CAD build for the part. Positions are in the model's coordinates, mm. A direction names the side the tool comes from. Round coordinates to 2 decimals unless told otherwise and drop trailing zeros. Write each loop counter-clockwise with the first axis right and the second up, starting at its lowest first coordinate (ties: lowest second). Pieces come first, ordered by that corner, then holes. Notation, with made-up numbers: M 82.5,35 L 114.5,35 A27 ccw 114.5,59 Z; hole C 71,-19.75 d10. An arc over 180 degrees is marked long. Write each question's results on one line, items separated by ' | '. Start each with the question number.
```python
from build123d import *

# Parameters (mm, degrees)
SKETCH1_R           = 2.1
SKETCH1_R_2         = 2.85
BOSS_EXTRUDE1_DEPTH = 9
CUT_EXTRUDE1_DEPTH  = 4
SKETCH10_W          = 28.2
SKETCH10_H          = 42
CUT_EXTRUDE8_DEPTH  = 5
SKETCH11_R          = 2.1
CUT_EXTRUDE9_DEPTH  = 5
CUT_EXTRUDE2_DEPTH  = 2
SKETCH5_R           = 2.85
CUT_EXTRUDE3_DEPTH  = 8
SKETCH7_W           = 75.2
SKETCH7_H           = 40.5
CUT_EXTRUDE5_DEPTH  = 6
SKETCH12_R          = 2.85
CUT_EXTRUDE10_DEPTH = 10
CUT_EXTRUDE11_DEPTH = 0.9
FILLET1_R           = 2
FILLET2_R           = 2
FILLET3_R           = 2


with BuildPart() as part:
    # Sketch1 → Boss-Extrude1 (new body)
    with BuildSketch(Plane(origin=(0, 0, 0), x_dir=(1, 0, 0), z_dir=(0, 1, 0))):
        Polygon((76.6, 0), (125, 0), (125, 150), (0, 150), (0, 0), (48.4, 0), (48.4, -15), (76.6, -15), align=None)
        with Locations((6.1, 127.9)):
            Circle(SKETCH1_R, mode=Mode.SUBTRACT)
        with Locations((6.1, 111.9)):
            Circle(SKETCH1_R, mode=Mode.SUBTRACT)
        with Locations((118.9, 127.9)):
            Circle(SKETCH1_R, mode=Mode.SUBTRACT)
        with Locations((118.9, 111.9)):
            Circle(SKETCH1_R, mode=Mode.SUBTRACT)
        with Locations((118.9, 22.1)):
            Circle(SKETCH1_R, mode=Mode.SUBTRACT)
        with Locations((118.9, 6.1)):
            Circle(SKETCH1_R, mode=Mode.SUBTRACT)
        with Locations((6.1, 6.1)):
            Circle(SKETCH1_R, mode=Mode.SUBTRACT)
        with Locations((6.1, 22.1)):
            Circle(SKETCH1_R, mode=Mode.SUBTRACT)
        with Locations((54.5, -8.9)):
            Circle(SKETCH1_R, mode=Mode.SUBTRACT)
        with Locations((70.5, -8.9)):
            Circle(SKETCH1_R, mode=Mode.SUBTRACT)
        with Locations((62.5, -0.9)):
            Circle(SKETCH1_R, mode=Mode.SUBTRACT)
        with Locations((102.5, 53)):
            Circle(SKETCH1_R_2, mode=Mode.SUBTRACT)
        with Locations((22.5, 69)):
            Circle(SKETCH1_R_2, mode=Mode.SUBTRACT)
        with Locations((102.5, 69)):
            Circle(SKETCH1_R_2, mode=Mode.SUBTRACT)
        with Locations((22.5, 53)):
            Circle(SKETCH1_R_2, mode=Mode.SUBTRACT)
    extrude(amount=BOSS_EXTRUDE1_DEPTH)

    # Sketch2 → Cut-Extrude1 (cut)
    with BuildSketch(Plane(origin=(0, 9, 0), x_dir=(1, 0, 0), z_dir=(0, 1, 0))):
        Polygon((76.6, -15), (76.6, 0), (76.6, 6.2), (48.4, 6.2), (48.4, 0), (48.4, -15), align=None)
    extrude(amount=-CUT_EXTRUDE1_DEPTH, mode=Mode.SUBTRACT)

    # Sketch10 → Cut-Extrude8 (cut)
    with BuildSketch(Plane(origin=(0, 0, 0), x_dir=(1, 0, 0), z_dir=(0, 1, 0))):
        with Locations((62.5, 6)):
            Rectangle(SKETCH10_W, SKETCH10_H)
    extrude(amount=CUT_EXTRUDE8_DEPTH, mode=Mode.SUBTRACT)

    # Sketch11 → Cut-Extrude9 (cut, through all)
    with BuildSketch(Plane.XZ.offset(-5)):
        with Locations((62.5, -16.6)):
            Circle(SKETCH11_R)
    extrude(amount=-CUT_EXTRUDE9_DEPTH, mode=Mode.SUBTRACT)

    # Sketch3 → Cut-Extrude2 (cut)
    with BuildSketch(Plane.XZ):
        Polygon((0, -56.45), (27, -56.45), (27, -46.45), (86.5, -46.45), (86.5, -56.45), (125, -56.45), (125, -95.45), (86.5, -95.45), (86.5, -105.45), (27, -105.45), (27, -95.45), (0, -95.45), align=None)
    extrude(amount=-CUT_EXTRUDE2_DEPTH, mode=Mode.SUBTRACT)

    # Sketch5 → Cut-Extrude3 (cut, through all)
    with BuildSketch(Plane.XZ.offset(-2)):
        with Locations((57.5, -52.45)):
            Circle(SKETCH5_R)
        with Locations((57.5, -99.45)):
            Circle(SKETCH5_R)
    extrude(amount=-CUT_EXTRUDE3_DEPTH, mode=Mode.SUBTRACT)

    # Sketch7 → Cut-Extrude5 (cut)
    with BuildSketch(Plane(origin=(0, 9, 0), x_dir=(1, 0, 0), z_dir=(0, 1, 0))):
        with Locations((62.5, 129.75)):
            Rectangle(SKETCH7_W, SKETCH7_H)
    extrude(amount=-CUT_EXTRUDE5_DEPTH, mode=Mode.SUBTRACT)

    # Sketch12 → Cut-Extrude10 (cut, through all)
    with BuildSketch(Plane(origin=(0, 9, 0), x_dir=(1, 0, 0), z_dir=(0, 1, 0))):
        with Locations((16.3, 145.05)):
            Circle(SKETCH12_R)
        with Locations((108.7, 145.05)):
            Circle(SKETCH12_R)
    extrude(amount=-CUT_EXTRUDE10_DEPTH, mode=Mode.SUBTRACT)

    # Sketch13 → Cut-Extrude11 (cut)
    with BuildSketch(Plane(origin=(0, 9, 0), x_dir=(1, 0, 0), z_dir=(0, 1, 0))):
        Polygon((24.9, 135), (8.9, 142), (8.9, 150), (24.9, 150), align=None)
        Polygon((100.1, 150), (100.1, 135), (116.1, 142), (116.1, 150), align=None)
    extrude(amount=-CUT_EXTRUDE11_DEPTH, mode=Mode.SUBTRACT)

    # Fillet1
    fillet1_edges = [part.edges().sort_by_distance(p)[0] for p in [
        (0, 4.5, -150),
        (125, 4.5, -150),
        (125, 4.5, 0),
        (0, 4.5, 0),
        (76.6, 7, -6.2),
        (48.4, 7, -6.2),
    ]]
    fillet(fillet1_edges, radius=FILLET1_R)

    # Fillet2
    fillet2_edges = [part.edges().sort_by_distance(p)[0] for p in [
        (76.6, 4.5, 0),
        (48.4, 4.5, 0),
    ]]
    fillet(fillet2_edges, radius=FILLET2_R)

    # Fillet3
    fillet3_edges = [part.edges().sort_by_distance(p)[0] for p in [
        (24.9, 6, -109.5),
        (24.9, 5.55, -150),
        (100.1, 5.55, -150),
        (100.1, 6, -109.5),
        (8.9, 8.55, -150),
        (8.9, 8.55, -142),
        (24.9, 8.55, -135),
        (100.1, 8.55, -135),
        (116.1, 8.55, -142),
        (116.1, 8.55, -150),
    ]]
    fillet(fillet3_edges, radius=FILLET3_R)


solid = part.part
```
1) Saw through at A-A, the plane z = -69. Write the cut outline in (x, y), plus the area to 3 significant figures.
2) Drop a flat-ended pin along its axis: pin 1 Ø2.5 at (x, y) = (65, 3.5) entering from +Z. Give the stop position or say it passes through.
3) Wall check: line 1 along Z through (x, y) = (102.5, 7.5); line 2 along X through (y, z) = (4.25, -127.9); line 3 along Z through (x, y) = (57.5, 7.25). Give the ranges that are in metal, low to high. Write a range as from..to.
4) 3-axis set-ups, long thin cutter, end or side, ignore diameter. For faces 1 (the face through (100.399, 5.451, -70.926)), 2 (the face through (63, 7, -6.2)), 3 (the face through (100.1, 6, -129)): which of +Z, -Z, +X, -X, +Y, -Y reach the whole face in a straight line?
5) Saw through at C-C, the plane z = -16.6. Write the cut outline in (x, y).
6) Pull direction X, two halves, no side cores. Call faces 4 (the face through (0, 4, -76)), 5 (the face through (62, 9, -59)), 6 (the face through (107, 8.1, -142)): pulls with the +X half, pulls with the -X half, needs draft (parallel to the pull), parting line crosses it, or undercut.
7) Saw through at B-B, the plane x = 62.5. Write the cut outline in (y, z).
8) Saw through at D-D, the plane x = 40. Write the cut outline in (y, z), plus the area to 3 significant figures.
Filled sheet:
1) outline: M 0,2 L 19.65,2 L 19.65,9 L 0,9 Z; M 25.35,2 L 99.65,2 L 99.65,9 L 25.35,9 Z; M 105.35,2 L 125,2 L 125,9 L 105.35,9 Z | area: 795 mm^2
2) pin 1: stops at z = -27
3) line 1: z = -150..-71.85, -66.15..-55.85, -50.15..0 | line 2: x = 0..4, 8.2..24.9, 100.1..116.8, 121..125 | line 3: z = -109.5..-102.3, -96.6..-55.3, -49.6..-6.2
4) face 1: +Y, -Y | face 2: +Z, +Y, -Y | face 3: -Z, +Y
5) outline: M 0,0 L 48.4,0 L 48.4,5 L 60.4,5 L 60.4,9 L 0,9 Z; M 64.6,5 L 76.6,5 L 76.6,0 L 125,0 L 125,9 L 64.6,9 Z
6) face 4: pulls with the -X half | face 5: needs draft | face 6: undercut
7) outline: M 0,-150 L 3,-150 L 3,-109.5 L 9,-109.5 L 9,-18.7 L 5,-18.7 L 5,-27 L 0,-27 L 0,-46.45 L 2,-46.45 L 2,-105.45 L 0,-105.45 Z; M 5,-14.5 L 9,-14.5 L 9,-6.2 L 5,-6.2 Z
8) outline: M 0,-150 L 3,-150 L 3,-109.5 L 9,-109.5 L 9,0 L 0,0 L 0,-46.45 L 2,-46.45 L 2,-105.45 L 0,-105.45 Z | area: 989 mm^2
